Autodesk Inventor part; units mm, degrees
ref_plane "YZ Plane" through (0, 0, 0) normal (1, 0, 0) x (0, 1, 0)
ref_plane "XZ Plane" through (0, 0, 0) normal (0, 1, 0) x (-1, 0, 0)
ref_plane "XY Plane" through (0, 0, 0) normal (0, 0, 1) x (1, 0, 0)
sketch "Sketch1" plane through (0, 0, 0) normal (0, 0, 1) x (1, 0, 0)
  line L0 (0, 0) -> (8.255, 0)
  line L1 (8.255, 0) -> (8.255, -8.255)
  line L2 (8.255, -8.255) -> (0, -8.255)
  line L3 (0, -8.255) -> (0, 0)
  dimension "d0" = 8.255
  dimension "d1" = 8.255
extrude "Extrusion1" add sketch "Sketch1" along normal blind 3.175
sketch "Sketch2" plane through (0, 0, 3.175) normal (0, 0, 1) x (1, 0, 0)
  circle A0 centre (4.1275, -4.1275) radius 3.81
  line L0 (0, 0) -> (0, -8.255)
  line L1 (8.255, 0) -> (0, 0)
  dimension "d4" = 7.62
  dimension "d5" = 4.1275
  dimension "d6" = 4.1275
extrude "Extrusion2" add sketch "Sketch2" along normal blind 1.905
properties part number "CameraLens" material "ABS Plastic"
The model under review builds one solid part; all positions refer to its coordinate system, in mm. A direction names the side the tool comes from. Round coordinates to 2 decimals unless told otherwise and drop trailing zeros. Order: outer loops, then holes, each group sorted by start corner. A loop starts at its lowest first (then second) coordinate and runs counter-clockwise, first axis right, second up. Notation, with made-up numbers: (54, 5.5) -> (61, 5.5) arc R8 cw to (61, 20.5) -> close; hole circle Ø8 at (6.5, 25). An arc over 180 degrees is marked (long way). Write item = value, one per line. Start each with the question number.
Item 1: For faces 1 (the face through (7.762, -5.272, 4.114)), 2 (the face through (4, 0, 2)), list the 3-axis set-ups (+Z, -Z, +X, -X, +Y, -Y) from which the entire face can be reached by the end or side of a thin tool; tool diameter is ignored.
Item 2: Consider section C-C on z = 4.05. Write out the cut boundary in (x, y).
Item 3: Consider section B-B on x = 7.5. Write out the cut boundary in (y, z) (3 decimals).
Item 4: Consider section A-A on y = -7.5. Write out the cut boundary in (x, z) (3 decimals), plus the area to 3 significant figures.
Item 5: For line 1 along X through (y, z) = (-4, 4.5); line 2 along Y through (x, z) = (4.25, 3.6); line 3 along Z through (x, y) = (6.75, -1.25) (3 decimals), list the stretches that pass through material, from the lowest coordinate up.
Conclusion:
q1.face_1 = +Z
q1.face_2 = +Z, -Z, +X, -X, +Y
q2.outline = circle Ø7.62 at (4.13, -4.13)
q3.outline = (-8.255, 0) -> (0, 0) -> (0, 3.175) -> (-2.355, 3.175) -> (-2.355, 5.08) -> (-5.9, 5.08) -> (-5.9, 3.175) -> (-8.255, 3.175) -> close
q4.outline = (0, 0) -> (8.255, 0) -> (8.255, 3.175) -> (5.9, 3.175) -> (5.9, 5.08) -> (2.355, 5.08) -> (2.355, 3.175) -> (0, 3.175) -> close
q4.area = 33.0 mm2
q5.line_1 = 0.32 to 7.94
q5.line_2 = -7.94 to -0.32
q5.line_3 = 0 to 3.175
